Check sheet for the modelled part. Datum: model origin and axes. Units: mm. A direction names the side the tool comes from. Give positions to 0.01 mm unless a question says otherwise; leave off trailing zeros. Loops run counter-clockwise (first coordinate to the right, second up) from the corner with the lowest first, then second, coordinate; pieces in that order, holes last. Notation, with made-up numbers: (54.25, 71) - (111.25, 71) arc R14 cw to (111.25, 81) - close; hole circle Ø11 at (-15.5, 4). An arc over 180 degrees is marked (long way). Use CSV: the item, a comma, the result in double quotes.
from build123d import *

# Parameters (mm, degrees)
F0_R                   = 28.5496
F1_DEPTH               = 38.1
F2_W                   = 20.32
F2_H                   = 22.1844250173
F2_H_2                 = 21.4777487576
F3_DEPTH               = 38.1
F3_DEPTH_BACK          = 38.1
F4_W                   = 45.6145062673
F4_H                   = 38.1
F5_DEPTH               = 25.4
F5_DEPTH_BACK          = 25.4
F7_D                   = 9.525
F7_DEPTH               = 25.4
F7_CBORE_D             = 9.525
F7_CBORE_DEPTH         = 6.35
F7_TIP                 = 2.8615986981
F9_D                   = 9.525
F9_DEPTH               = 25.4
F9_CBORE_D             = 9.525
F9_CBORE_DEPTH         = 6.35
F9_TIP                 = 2.8615986981
F12_D                  = 3.175
F12_DEPTH              = 25.4
F12_CBORE_D            = 3.175
F12_CBORE_DEPTH        = 6.35
F12_TIP                = 0.9538662327
F12_ON_F11_D           = 3.175
F12_ON_F11_DEPTH       = 25.4
F12_ON_F11_CBORE_D     = 3.175
F12_ON_F11_CBORE_DEPTH = 6.35
F12_ON_F11_TIP         = 0.9538662327
F13_R                  = 28.5496
F14_DEPTH              = 6.35
F15_R                  = 6.35
F16_DEPTH              = 25.4
F17_R                  = 25.4
F17_R_2                = 6.35
F18_DEPTH              = 10.16


with BuildPart() as f1:
    # F0 (on Right) → F1 (new body)
    with BuildSketch(Plane.YZ):
        Circle(F0_R)
    extrude(amount=F1_DEPTH)

    # F2 (on Front) → F3 (cut, two sides)
    with BuildSketch(Plane.XZ) as f3_sk:
        with Locations((29.21, 20.6172125086)):
            Rectangle(F2_W, F2_H)
        with Locations((29.21, -20.2638743788)):
            Rectangle(F2_W, F2_H_2)
    extrude(amount=-F3_DEPTH, mode=Mode.SUBTRACT)
    extrude(f3_sk.sketch, amount=F3_DEPTH_BACK, mode=Mode.SUBTRACT)

    # F4 (on Top) → F5 (cut, two sides)
    with BuildSketch(Plane.XY) as f5_sk:
        with Locations((41.8572531337, 0)):
            Rectangle(F4_W, F4_H)
    extrude(amount=-F5_DEPTH, mode=Mode.SUBTRACT)
    extrude(f5_sk.sketch, amount=F5_DEPTH_BACK, mode=Mode.SUBTRACT)

    # F7
    with Locations(Plane.XZ.offset(-19.05)):
        with Locations((28.575, 0)):
            CounterBoreHole(F7_D / 2, F7_CBORE_D / 2, F7_CBORE_DEPTH, depth=F7_DEPTH)
            with Locations((0, 0, -(F7_DEPTH + F7_TIP / 2))):  # 118° drill point
                Cone(0, F7_D / 2, F7_TIP, mode=Mode.SUBTRACT)

    # F9
    with Locations(Plane(origin=(0, -19.05, 0), x_dir=(-1, 0, 0), z_dir=(0, 1, 0))):
        with Locations((-28.575, 0)):
            CounterBoreHole(F9_D / 2, F9_CBORE_D / 2, F9_CBORE_DEPTH, depth=F9_DEPTH)
            with Locations((0, 0, -(F9_DEPTH + F9_TIP / 2))):  # 118° drill point
                Cone(0, F9_D / 2, F9_TIP, mode=Mode.SUBTRACT)

    # F12
    with Locations(Plane.XY.offset(9.525)):
        with Locations((28.575, 22.9819130483)):
            CounterBoreHole(F12_D / 2, F12_CBORE_D / 2, F12_CBORE_DEPTH, depth=F12_DEPTH)
            with Locations((0, 0, -(F12_DEPTH + F12_TIP / 2))):  # 118° drill point
                Cone(0, F12_D / 2, F12_TIP, mode=Mode.SUBTRACT)

    # F12 on F11
    with Locations(Plane.XY.offset(9.525)):
        with Locations((28.575, -22.9819130483)):
            CounterBoreHole(F12_ON_F11_D / 2, F12_ON_F11_CBORE_D / 2, F12_ON_F11_CBORE_DEPTH, depth=F12_ON_F11_DEPTH)
            with Locations((0, 0, -(F12_ON_F11_DEPTH + F12_ON_F11_TIP / 2))):  # 118° drill point
                Cone(0, F12_ON_F11_D / 2, F12_ON_F11_TIP, mode=Mode.SUBTRACT)

    # F13 (on face) → F14 (join)
    with BuildSketch(Plane(origin=(0, 0, 0), x_dir=(0, -1, 0), z_dir=(-1, 0, 0))):
        Circle(F13_R)
    extrude(amount=F14_DEPTH)

    # F15 (on face) → F16 (join)
    with BuildSketch(Plane(origin=(-6.35, 0, 0), x_dir=(0, -1, 0), z_dir=(-1, 0, 0))):
        Circle(F15_R)
    extrude(amount=F16_DEPTH)

    # F17 (on face) → F18 (cut)
    with BuildSketch(Plane(origin=(-6.35, 0, 0), x_dir=(0, -1, 0), z_dir=(-1, 0, 0))):
        Circle(F17_R)
        Circle(F17_R_2, mode=Mode.SUBTRACT)
    extrude(amount=-F18_DEPTH, mode=Mode.SUBTRACT)


solid = f1.part
1. Scan lines: line 1 along Z through (x, y) = (1.25, 0); line 2 along Y through (x, z) = (35.5, 1); line 3 along X through (y, z) = (-2, -11). Record each from-to range of solid material in increasing order.
Completed:
line 1,"z = -28.55 to -25.4, -6.35 to 6.35, 25.4 to 28.55"
line 2,"y = -28.53 to -19.05, 19.05 to 28.53"
line 3,"x = 3.81 to 19.05"
2. Sectioned sample at A-A, the plane z = 0. Record the boundary of the cut face in (x, y), and give its area (3 significant figures).
Completed:
outline,"(-31.75, -6.35) - (3.81, -6.35) - (3.81, -25.4) - (-6.35, -25.4) - (-6.35, -28.55) - (23.81, -28.55) - (23.81, -19.05) - (19.05, -19.05) - (19.05, 19.05) - (23.81, 19.05) - (23.81, 28.55) - (-6.35, 28.55) - (-6.35, 25.4) - (3.81, 25.4) - (3.81, 6.35) - (-31.75, 6.35) - close; (33.34, -28.55) - (38.1, -28.55) - (38.1, -19.05) - (33.34, -19.05) - close; (33.34, 19.05) - (38.1, 19.05) - (38.1, 28.55) - (33.34, 28.55) - close"
area,"1,570 mm²"
3. Go/stop test with flat-tipped pins: pin 1 Ø4 at (x, y) = (27.5, 22.5) entering from -Z (3 decimals); pin 2 Ø1 at (x, z) = (-15, 2.5) entering from -Y; pin 3 Ø4 at (x, y) = (33, 22) entering from +Z (3 decimals); pin 4 Ø9.5 at (x, z) = (25.5, 0.5) entering from -Y. Record where each tip stops, or that it passes through.
Completed:
pin 1,"stops at z = -9.525"
pin 2,"stops at y = -6.03"
pin 3,"stops at z = 9.525"
pin 4,"stops at y = -28.55"
4. Sectioned sample at D-D, the plane x = 5.5. Record the boundary of the cut face in (y, z), and give its area (3 significant figures).
Completed:
outline,"circle Ø57.1 at (0, 0)"
area,"2,560 mm²"
5. Release check for a two-part mould opening along Y. For faces 4 (the face through (27.722, -21.643, -7.043)), 5 (the face through (-6.35, 26, -2)) record: released by +Y, released by -Y, zero draft, split by the parting line, or undercut.
Completed:
face 4,"undercut"
face 5,"zero draft"
6. Sectioned sample at B-B, the plane x = 22. Record the boundary of the cut face in (y, z) (3 decimals), and give its area (3 significant figures).
Completed:
outline,"(-26.914, -9.525) - (-19.05, -9.525) - (-19.05, 9.525) - (-26.914, 9.525) arc R28.55 ccw to start; (19.05, -9.525) - (26.914, -9.525) arc R28.55 ccw to (26.914, 9.525) - (19.05, 9.525) - close"
area,"341 mm²"
7. Set-up check for faces 1 (the face through (28, 21, 9.525)), 2 (the face through (26.3, -19.05, 4.4)), 3 (the face through (28, -21, -9.525)): record each of +Z, -Z, +X, -X, +Y, -Y from which the full face is reachable in a straight line by a thin tool's end or side.
Completed:
face 1,"+Z, +X, +Y, -Y"
face 2,"+Z, -Z, +X"
face 3,"-Z, +X, +Y, -Y"
8. Sectioned sample at C-C, the plane y = 0. Record the boundary of the cut face in (x, z).
Completed:
outline,"(-31.75, -6.35) - (3.81, -6.35) - (3.81, -25.4) - (-6.35, -25.4) - (-6.35, -28.55) - (19.05, -28.55) - (19.05, 28.55) - (-6.35, 28.55) - (-6.35, 25.4) - (3.81, 25.4) - (3.81, 6.35) - (-31.75, 6.35) - close"
